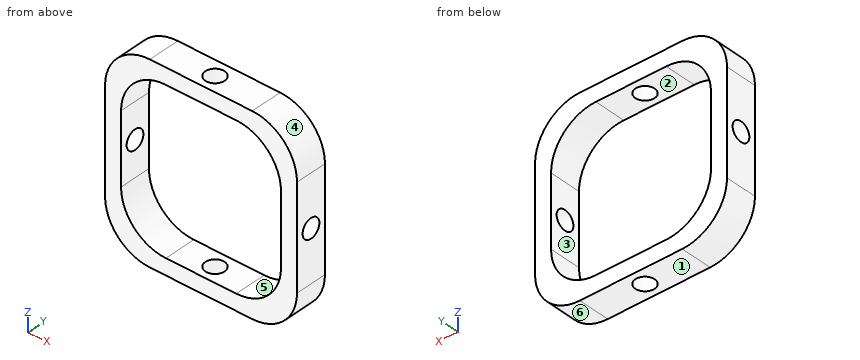
from build123d import *

# Parameters (mm, degrees)
CROQUIS1_W                 = 30
CROQUIS1_H                 = 30
CROQUIS1_W_2               = 25
CROQUIS1_H_2               = 25
SALIENTE_EXTRUIR1_DEPTH    = 5
CROQUIS2_R                 = 1.5
CORTAR_EXTRUIR1_DEPTH      = 1
CORTAR_EXTRUIR1_DEPTH_BACK = 31
CROQUIS3_R                 = 1.5
CORTAR_EXTRUIR2_DEPTH      = 1
CORTAR_EXTRUIR2_DEPTH_BACK = 31
REDONDEO1_R                = 7


with BuildPart() as part:
    # Croquis1 → Saliente-Extruir1 (new body)
    with BuildSketch(Plane(origin=(0, 0, 0), x_dir=(1, 0, 0), z_dir=(0, 1, 0))):
        Rectangle(CROQUIS1_W, CROQUIS1_H)
        Rectangle(CROQUIS1_W_2, CROQUIS1_H_2, mode=Mode.SUBTRACT)
    extrude(amount=SALIENTE_EXTRUIR1_DEPTH)

    # Croquis2 → Cortar-Extruir1 (cut, two sides)
    with BuildSketch(Plane.XY.offset(15)) as cortar_extruir1_sk:
        with Locations((0, 2.5)):
            Circle(CROQUIS2_R)
    extrude(amount=CORTAR_EXTRUIR1_DEPTH, mode=Mode.SUBTRACT)
    extrude(cortar_extruir1_sk.sketch, amount=-CORTAR_EXTRUIR1_DEPTH_BACK, mode=Mode.SUBTRACT)

    # Croquis3 → Cortar-Extruir2 (cut, two sides)
    with BuildSketch(Plane.ZY.offset(15)) as cortar_extruir2_sk:
        with Locations((0, 2.5)):
            Circle(CROQUIS3_R)
    extrude(amount=CORTAR_EXTRUIR2_DEPTH, mode=Mode.SUBTRACT)
    extrude(cortar_extruir2_sk.sketch, amount=-CORTAR_EXTRUIR2_DEPTH_BACK, mode=Mode.SUBTRACT)

    # Redondeo1
    redondeo1_edges = [part.edges().sort_by_distance(p)[0] for p in [
        (-12.5, 2.5, -12.5),
        (-12.5, 2.5, 12.5),
        (12.5, 2.5, 12.5),
        (12.5, 2.5, -12.5),
        (15, 2.5, 15),
        (-15, 2.5, 15),
        (-15, 2.5, -15),
        (15, 2.5, -15),
    ]]
    fillet(redondeo1_edges, radius=REDONDEO1_R)


solid = part.part
For this review, take the finished solid that the model builds, in its own axes (mm). Face numbers are marked on the shaded views. A direction names the side the tool comes from. Give positions to 0.01 mm unless a question says otherwise; leave off trailing zeros. Order: outer loops, then holes, each group sorted by start corner. A loop starts at its lowest first (then second) coordinate and runs counter-clockwise, first axis right, second up. Notation, with made-up numbers: M 17,36 L 61,36 A17 cw 61,55 Z; hole C 21.25,59.5 d3. An arc over 180 degrees is marked long. Answer in a Markdown table with one row per item. Add a question column.
(1) For the marked faces 5 and 6, list the 3-axis set-ups (+Z, -Z, +X, -X, +Y, -Y) from which the entire face can be reached by the end or side of a thin tool; tool diameter is ignored.
(2) Consider section D-D on z = -6.25. State the section outline as (x, y) points, and give its area (3 significant figures).
(3) Consider section B-B on y = 2.5. Give the number of separate pieces and of enclosed holes in the cut face, and give its area (3 significant figures).
(4) Wall thickness on probe 1 along Y at (x, z) = (-13.85, 0); probe 2 along X at (y, z) = (4.25, -3): over which ranges is each line inside the solid? List them lowest first. Write a range as [from, to].
(5) Consider section A-A on x = 0. State the section outline as (y, z) points, and give its area (3 significant figures).
(6) Consider section C-C on z = 0. State the section outline as (x, y) points.
(7) Mouldability with a two-part tool opening along Z and no side actions: class the marked faces 1, 2, 3 and 4 as +Z half, -Z half, draft (parallel to the pull), parting line (faces both ways), or undercut.
(8) For pin 1 (2.5 mm diameter, centred on y = 2.5, z = 0, fed in from -X); pin 2 (1.5 mm diameter, centred on x = 11.5, y = 3, fed in from +Z), all flat-tipped, find the tip position at first contact; note any pin that passes through.
Evaluation:
| question | item | result |
|---|---|---|
| 1 | face 5 | +Y, -Y |
| 1 | face 6 | -Z, +X, +Y, -Y |
| 2 | outline | M -15,0 L -12.46,0 L -12.46,5 L -15,5 Z; M 12.46,0 L 15,0 L 15,5 L 12.46,5 Z |
| 2 | area | 25.4 mm^2 |
| 3 | separate pieces | 4 |
| 3 | enclosed holes | 0 |
| 3 | area | 245 mm^2 |
| 4 | probe 1 | y = [0, 1], [4, 5] |
| 4 | probe 2 | x = [-15, -12.5], [12.5, 15] |
| 5 | outline | M 0,-15 L 1,-15 L 1,-12.5 L 0,-12.5 Z; M 0,12.5 L 1,12.5 L 1,15 L 0,15 Z; M 4,-15 L 5,-15 L 5,-12.5 L 4,-12.5 Z; M 4,12.5 L 5,12.5 L 5,15 L 4,15 Z |
| 5 | area | 10.0 mm^2 |
| 6 | outline | M -15,0 L -12.5,0 L -12.5,1 L -15,1 Z; M -15,4 L -12.5,4 L -12.5,5 L -15,5 Z; M 12.5,0 L 15,0 L 15,1 L 12.5,1 Z; M 12.5,4 L 15,4 L 15,5 L 12.5,5 Z |
| 7 | face 1 | -Z half |
| 7 | face 2 | undercut |
| 7 | face 3 | undercut |
| 7 | face 4 | +Z half |
| 8 | pin 1 | passes through |
| 8 | pin 2 | stops at z = 14.44 |
